The model under review builds one solid part; all positions refer to its coordinate system, in mm. Face numbers are marked on the shaded views. Round coordinates to 2 decimals unless told otherwise and drop trailing zeros. Write each loop counter-clockwise with the first axis right and the second up, starting at its lowest first coordinate (ties: lowest second). Pieces come first, ordered by that corner, then holes. Notation, with made-up numbers: (-27, 10) -> (6, 10) arc R29 cw to (6, 44) -> close; hole circle Ø2 at (60.5, -5). An arc over 180 degrees is marked (long way). Use CSV: the item, a comma, the result in double quotes. Start each with the question number.
1) For pin 1 Ø5 at (x, y) = (1.5, 47) entering from -Z; pin 2 Ø4 at (x, y) = (-12, 34) entering from +Z; pin 3 Ø3 at (y, z) = (48, 39) entering from +X; pin 4 Ø6 at (y, z) = (61, 23) entering from -X, all flat-tipped, find the tip position at first contact; note any pin that passes through.
2) Take a section at A-A, the plane y = 34. Give the boundary of the cut face in (x, z), then the cut area to 3 significant figures.
3) Take a section at B-B, the plane x = -12. Give the boundary of the cut face in (y, z), then the cut area to 3 significant figures.
4) Take a section at C-C, the plane y = 11.5. Give the boundary of the cut face in (x, z), then the cut area to 3 significant figures.
5) Wall thickness on probe 1 along X at (y, z) = (86, 1.95); probe 2 along Y at (x, z) = (-12, 2.2); probe 3 along X at (y, z) = (60.5, 11.5): over which ranges is each line inside the solid? List them lowest first. Write a range as [from, to].
6) Mouldability with a two-part tool opening along X and no side actions: class the marked faces 1, 2 and 3 as released by +X, released by -X, zero draft, split by the parting line, or undercut.
Autodesk Inventor part; units mm, degrees
ref_plane "YZ Plane" through (0, 0, 0) normal (1, 0, 0) x (0, 1, 0)
ref_plane "XZ Plane" through (0, 0, 0) normal (0, 1, 0) x (-1, 0, 0)
ref_plane "XY Plane" through (0, 0, 0) normal (0, 0, 1) x (1, 0, 0)
sketch "Sketch1" plane through (0, 0, 0) normal (0, 0, 1) x (1, 0, 0)
  line L0 (-8, 0) -> (0, 0)
  line L1 (0, 0) -> (0, 120)
  line L2 (0, 120) -> (-8, 120)
  line L3 (-8, 120) -> (-8, 0)
  line L4 (0, 34) -> (-16, 34) construction
  line L5 (-8, 30) -> (-12, 30)
  line L6 (-12, 38) -> (-8, 38)
  arc A0 (-12, 38) -> (-12, 30) centre (-12, 34) ccw
  line L7 (0, 86) -> (-16, 86) construction
  line L8 (-8, 82) -> (-12, 82)
  line L9 (-12, 90) -> (-8, 90)
  arc A1 (-12, 90) -> (-12, 82) centre (-12, 86) ccw
  circle A2 centre (-12, 34) radius 1.75
  circle A3 centre (-12, 86) radius 1.75
  line L10 (0, 60) -> (-8, 60)
  point P0 (-8, 34)
  point P1 (-8, 86)
  dimension "d0" = 8
  dimension "d1" = 120
  dimension "d2" = 52
  dimension "d3" = 3.5
  dimension "d4" = 3.5
  dimension "d5" = 4
  dimension "d6" = 4
  dimension "d7" = 4
extrude "Extrusion1" add sketch "Sketch1" along normal blind 4
sketch "Sketch2" plane through (-8, 0, 0) normal (0, -1, 0) x (1, 0, 0)
  line L0 (0, 0) -> (8, 0)
  line L1 (8, 0) -> (8, 4)
  line L2 (0, 4) -> (8, 4)
  line L3 (0, 0) -> (0, 4)
  line L4 (8, 4) -> (8, 44)
  arc A0 (88.2833, 74.4337) -> (8, 44) centre (63, 20.0208) ccw
  arc A1 (88.2833, 77.7249) -> (0, 20.0208) centre (63, 20.0208) ccw
  line L5 (88.2833, 77.7249) -> (88.2833, 74.4337)
  line L6 (0, 4) -> (0, 20.0208)
  dimension "d10" = 40
  dimension "d11" = 60
  dimension "d20" = 63
  dimension "d22" = 3.2912
extrude "Extrusion2" add sketch "Sketch2" against normal up to surface (120 mm away) from surface at 0 contours L6 A1 L5 A0 L4 L2
fillet "Fillet1" radius 20 1 edges at (0, 60, 44)
fillet "Fillet2" radius 20 4 edges at (-8, 38, 2) (-8, 90, 2) (-8, 82, 2) (-8, 30, 2)
fillet "Fillet3" radius 1.5 12 edges at (-8, 120, 10.0104) (20.5315, 120, 72.7553) (0.6351, 120, 44.3858) (0, 120, 19.6929) (36.3979, 120, 77.0643) (80.2833, 60, 77.7249) (80.2833, 60, 74.4337) (-8, 0, 10.0104) (20.5315, 0, 72.7553) (0.6351, 0, 44.3858) (0, 0, 19.6929) (36.3979, 0, 77.0643)
fillet "Fillet4" radius 2 2 edges at (-8, 34, 4) (-8, 86, 4)
properties part number "tunel.viento"
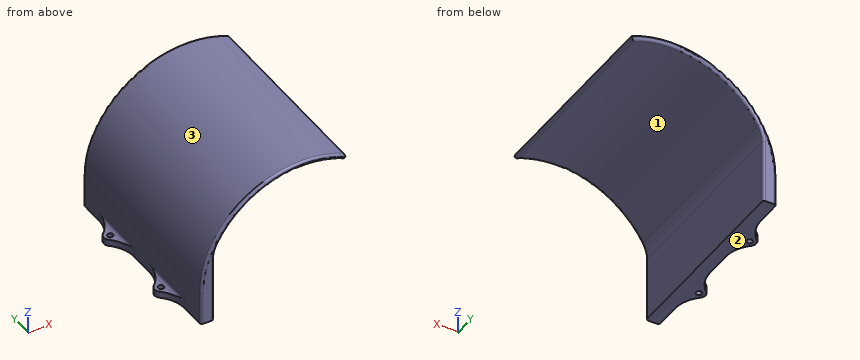
Values found:
1,pin 1,"z = 0"
1,pin 2,"z = 4"
1,pin 3,"x = 0.03"
1,pin 4,"x = -8"
2,outline,"(-16, 0) -> (-13.75, 0) -> (-13.75, 4) -> (-16, 4) -> close; (-10.25, 0) -> (0, 0) -> (0, 39.39) arc R20 cw to (2.5, 49.07) arc R60 cw to (78.2, 75.35) arc R1.5 ccw to (80.28, 76.74) arc R1.5 ccw to (79.36, 78.12) arc R63 ccw to (-8, 20.02) -> (-8, 6) arc R2 cw to (-10, 4) -> (-10.25, 4) -> close"
2,area,"628 mm²"
3,outline,"(28.11, 0) -> (32.25, 0) -> (32.25, 4) -> (28.11, 4) -> close; (35.75, 0) -> (39.89, 0) -> (39.89, 4) -> (35.75, 4) -> close; (80.11, 0) -> (84.25, 0) -> (84.25, 4) -> (80.11, 4) -> close; (87.75, 0) -> (91.89, 0) -> (91.89, 4) -> (87.75, 4) -> close"
3,area,"66.2 mm²"
4,outline,"(-8, 0) -> (0, 0) -> (0, 39.39) arc R20 cw to (2.5, 49.07) arc R60 cw to (78.2, 75.35) arc R1.5 ccw to (80.28, 76.74) arc R1.5 ccw to (79.36, 78.12) arc R63 ccw to (-8, 20.02) -> close"
4,area,"609 mm²"
5,probe 1,"[-16, -13.75], [-10.25, 0]"
5,probe 2,"[28.11, 32.25], [35.75, 39.89], [80.11, 84.25], [87.75, 91.89]"
5,probe 3,"[-8, 0]"
6,face 1,"undercut"
6,face 2,"zero draft"
6,face 3,"split by the parting line"
